from build123d import *

# Parameters (mm, degrees)
BOSS_EXTRUDE4_DEPTH = 15
BOSS_EXTRUDE5_REACH = 42.927
SKETCH8_R           = 3.25
CUT_EXTRUDE1_DEPTH  = 41.926763896


with BuildPart() as part:
    # Sketch2 → Boss-Extrude4 (new, symmetric)
    with BuildSketch(Plane.XY):
        with BuildLine():
            Line((-22.5, 0), (-35, 0))
            Line((-35, 0), (-35, 3))
            Line((-35, 3), (-25.322914524, 3))
            ThreePointArc((-25.322914524, 3), (0, 25.5), (25.322914524, 3))
            Line((25.322914524, 3), (35, 3))
            Line((35, 3), (35, 0))
            Line((35, 0), (22.5, 0))
            ThreePointArc((22.5, 0), (0, 22.5), (-22.5, 0))
        make_face()
    extrude(amount=BOSS_EXTRUDE4_DEPTH, both=True)

    # Sketch5 → Boss-Extrude5 (add, up to next)
    with BuildSketch(Plane(origin=(0, 15, 0), x_dir=(1, 0, 0), z_dir=(0, 1, 0)), mode=Mode.PRIVATE) as boss_extrude5_sk1:
        with BuildLine():
            Line((-23.872753943, 6), (-13.872753943, 6))
            Line((-13.872753943, 6), (-13.872753943, -6))
            Line((-13.872753943, -6), (-23.872753943, -6))
            ThreePointArc((-23.872753943, -6), (-29.872753943, 0), (-23.872753943, 6))
        make_face()
    boss_extrude5_tool1 = extrude(boss_extrude5_sk1.sketch, amount=-BOSS_EXTRUDE5_REACH, mode=Mode.PRIVATE) - part.part
    boss_extrude5 = boss_extrude5_tool1.solids().sort_by_distance((-21.289897, 15, 0))[0]
    add(boss_extrude5)

    # Sketch8 → Cut-Extrude1 (cut, through all)
    with BuildSketch(Plane(origin=(0, 15, 0), x_dir=(1, 0, 0), z_dir=(0, 1, 0))):
        with Locations(Location((-23.872753943, 0, 0), (0, 0, 270))):
            Circle(SKETCH8_R)
    cut_extrude1 = extrude(amount=-CUT_EXTRUDE1_DEPTH, mode=Mode.SUBTRACT)

    # Mirror1: Boss-Extrude5 across plane
    add(boss_extrude5.mirror(Plane(origin=(0, 0, 0), x_dir=(0, 0, 1), z_dir=(1, 0, 0))))

    # Mirror2: Cut-Extrude1 across plane
    add(cut_extrude1.mirror(Plane(origin=(0, 0, 0), x_dir=(0, 0, 1), z_dir=(1, 0, 0))), mode=Mode.SUBTRACT)


solid = part.part
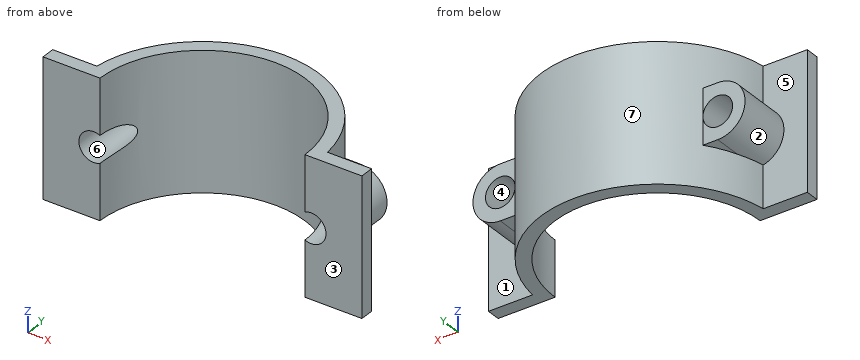
Here's how the part is built. I have some questions about the finished solid (model axes, mm). Face numbers are marked on the shaded views. A direction names the side the tool comes from. Give positions to 0.01 mm unless a question says otherwise; leave off trailing zeros. Write each loop counter-clockwise with the first axis right and the second up, starting at its lowest first coordinate (ties: lowest second). Pieces come first, ordered by that corner, then holes. Notation, with made-up numbers: (-33, 3) -> (-28, 3) arc R17 ccw to (-28, 13) -> close; hole circle Ø11 at (-4, 83). An arc over 180 degrees is marked (long way). Use one line per item in the form item = value. Start each with the question number.
1. On a 3-axis mill with a long thin cutter (end or side, diameter ignored), from which of +Z, -Z, +X, -X, +Y, -Y can I reach the whole of each face in a straight line? I mean the marked faces 1, 2 and 3. Say none if no direction works.
2. Imagine slicing it at C-C on z = -7.5. List the corners of the cut face in (x, y) for me, plus the area to 3 significant figures.
3. If I drill on L1, parallel to X at y = 11.5, z = 0; L2, parallel to X at y = 10.25, z = 0; L3, parallel to Y at x = 9, z = -4, over which ranges is the centre line in solid material (lowest first)?
4. Imagine slicing it at D-D on y = 13.5. List the corners of the cut face in (x, z) for me, plus the area to 3 significant figures.
5. Imagine slicing it at B-B on y = 20.75. List the corners of the cut face in (x, z) for me, plus the area to 3 significant figures.
6. Will these pins go through, and if not, where does the flat tip stop? pin 1 Ø5 at (x, z) = (-30, -1) entering from +Y; pin 2 Ø7.5 at (x, z) = (-23, -1) entering from +Y; pin 3 Ø1 at (y, z) = (7.5, 5) entering from +X.
7. Thinking about a two-plate mould opening in X: for the marked faces 4, 5, 6 and 7, which applies, +X half, -X half, draft (parallel to the pull), parting line (faces both ways), or undercut?
8. Imagine slicing it at A-A on z = -2. List the corners of the cut face in (x, y) for me, plus the area to 3 significant figures.
Entries:
q1.face_1 = +X, +Y
q1.face_2 = -X, +Y
q1.face_3 = +Z, -Z, +X, -X, -Y
q2.outline = (-35, 0) -> (-22.5, 0) arc R22.5 cw to (22.5, 0) -> (35, 0) -> (35, 3) -> (25.32, 3) arc R25.5 ccw to (-25.32, 3) -> (-35, 3) -> close
q2.area = 284 mm²
q3.L1 = -29.87 to -27.12, -20.62 to -19.34, 19.34 to 20.62, 27.12 to 29.87
q3.L2 = -29.87 to -27.12, -20.62 to -20.03, 20.03 to 20.62, 27.12 to 29.87
q3.L3 = 20.62 to 23.86
q4.outline = (-23.87, -6) -> (-21.63, -6) -> (-21.63, -15) -> (-18, -15) -> (-18, 15) -> (-21.63, 15) -> (-21.63, 6) -> (-23.87, 6) arc R6 ccw to start; (18, -15) -> (21.63, -15) -> (21.63, -6) -> (23.87, -6) arc R6 ccw to (23.87, 6) -> (21.63, 6) -> (21.63, 15) -> (18, 15) -> close; hole circle Ø6.5 at (-23.87, 0); hole circle Ø6.5 at (23.87, 0)
q4.area = 318 mm²
q5.outline = (-14.82, -15) -> (-8.7, -15) -> (-8.7, 15) -> (-14.82, 15) -> close; (8.7, -15) -> (14.82, -15) -> (14.82, 15) -> (8.7, 15) -> close
q5.area = 367 mm²
q6.pin_1 = 15
q6.pin_2 = 16.72
q6.pin_3 = 27.84
q7.face_4 = undercut
q7.face_5 = draft
q7.face_6 = undercut
q7.face_7 = parting line
q8.outline = (-35, 0) -> (-26.43, 0) -> (-26.43, 15) -> (-29.53, 15) -> (-29.53, 3) -> (-35, 3) -> close; (-21.31, 7.22) arc R22.5 cw to (21.31, 7.22) -> (21.31, 15) -> (20.62, 15) arc R25.5 ccw to (-20.62, 15) -> (-21.31, 15) -> close; (26.43, 0) -> (35, 0) -> (35, 3) -> (29.53, 3) -> (29.53, 15) -> (26.43, 15) -> close
q8.area = 284 mm²
